from build123d import *

# Parameters (mm, degrees)
F1_DEPTH  = 18
F2_R      = 2.1
F3_DEPTH  = 25
F4_START  = -9
F2_R_2    = 4.1
F4_DEPTH  = 16
F6_START  = -9
F5_R      = 4.1
F5_R_2    = 2.1
F6_DEPTH  = 16
F7_DEPTH  = 25
F8_R      = 1
F2_W      = 8
F2_H      = 4.2
F9_DEPTH  = 1.5
F5_W      = 4.2
F5_H      = 8
F10_DEPTH = 1.5
F11_R     = 0.5


with BuildPart() as f1:
    # F0 (on Front) → F1 (new body)
    with BuildSketch(Plane.XZ):
        Polygon((-30, 10), (-30, 0), (0, 0), (21.2132034356, 21.2132034356), (14.1421356237, 28.2842712475), align=None)
    extrude(amount=F1_DEPTH)

    # F2 (on face) → F3 (cut)
    with BuildSketch(Plane(origin=(0, 0, 0), x_dir=(1, 0, 0), z_dir=(0, 0, -1))):
        with Locations((-21, 9)):
            Circle(F2_R)
    extrude(amount=-F3_DEPTH, mode=Mode.SUBTRACT)

    # F2 (on face) → F4 (cut)
    with BuildSketch(Plane(origin=(0, 0, 0), x_dir=(1, 0, 0), z_dir=(0, 0, -1)).offset(F4_START)):
        with Locations((-21, 9)):
            Circle(F2_R_2)
        with Locations((-21, 9)):
            Circle(F2_R, mode=Mode.SUBTRACT)
    extrude(amount=-F4_DEPTH, mode=Mode.SUBTRACT)

    # F5 (on face) → F6 (cut)
    with BuildSketch(Plane(origin=(0, 0, 0), x_dir=(0, 1, 0), z_dir=(0.7071067812, 0, -0.7071067812)).offset(F6_START)):
        with Locations((-9, 21)):
            Circle(F5_R)
        with Locations((-9, 21)):
            Circle(F5_R_2, mode=Mode.SUBTRACT)
    extrude(amount=-F6_DEPTH, mode=Mode.SUBTRACT)

    # F5 (on face) → F7 (cut)
    with BuildSketch(Plane(origin=(0, 0, 0), x_dir=(0, 1, 0), z_dir=(0.7071067812, 0, -0.7071067812))):
        with Locations((-9, 21)):
            Circle(F5_R_2)
    extrude(amount=-F7_DEPTH, mode=Mode.SUBTRACT)

    # F8
    f8_edges = [f1.edges().sort_by_distance(p)[0] for p in [
        (-30, -9, 0),
        (-30, -9, 10),
        (21.213203, -9, 21.213203),
        (14.142136, -9, 28.284271),
        (-25.1, -8.999972, 12.029646),
    ]]
    fillet(f8_edges, radius=F8_R)

    # F2 (on face) → F9 (join)
    with BuildSketch(Plane(origin=(0, 0, 0), x_dir=(1, 0, 0), z_dir=(0, 0, -1))):
        with Locations((-7, 9)):
            Rectangle(F2_W, F2_H)
    extrude(amount=F9_DEPTH)

    # F5 (on face) → F10 (join)
    with BuildSketch(Plane(origin=(0, 0, 0), x_dir=(0, 1, 0), z_dir=(0.7071067812, 0, -0.7071067812))):
        with Locations((-9, 7)):
            Rectangle(F5_W, F5_H)
    extrude(amount=F10_DEPTH)

    # F11
    f11_edges = [f1.edges().sort_by_distance(p)[0] for p in [
        (-7, -6.9, 0),
        (-7, -6.9, -1.5),
        (-7, -11.1, -1.5),
        (-7, -11.1, 0),
        (4.949747, -11.1, 4.949747),
        (6.010408, -11.1, 3.889087),
        (6.010408, -6.9, 3.889087),
        (4.949747, -6.9, 4.949747),
    ]]
    fillet(f11_edges, radius=F11_R)


solid = f1.part
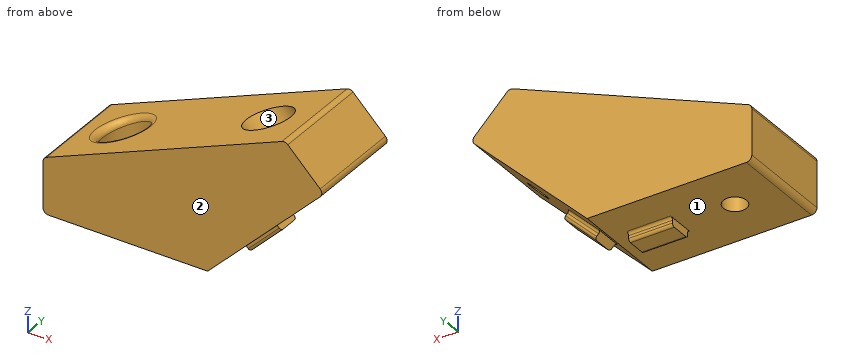
Geometry check sheet. Reference: the model listing, model coordinates, mm. Face numbers are marked on the shaded views. Give positions to 0.01 mm unless a question says otherwise; leave off trailing zeros. Loops run counter-clockwise (first coordinate to the right, second up) from the corner with the lowest first, then second, coordinate; pieces in that order, holes last. Notation, with made-up numbers: (-7.5, -20) -> (37.5, -20) arc R23 ccw to (37.5, 19) -> close; hole circle Ø10 at (80.5, -30.5). An arc over 180 degrees is marked (long way). Answer in a Markdown table with one row per item. Add a question column.
1) Cross-section at C-C on x = -1. Record the boundary of the cut face in (y, z), and give its area (3 significant figures).
2) Cross-section at A-A on z = 0.5. Record the boundary of the cut face in (x, y).
3) Gauge pin test, flat ends, axial feed: P1, Ø5.5, axis at x = -21, y = -9, coming from the -Z side; P2, Ø5, axis at x = -21, y = -9, coming from the +Z side; P3, Ø1, axis at y = -5.5, z = 23, coming from the +X side. Record the tip position at first contact, or that the pin passes through.
4) Draft check along Z on the marked faces 1, 2 and 3. Enter one of: pulls with the +Z half, pulls with the -Z half, needs draft (parallel to the pull), parting line crosses it, or undercut.
5) Material ranges on probe 1 along Y at (x, z) = (-21, 2.75); probe 2 along Y at (x, z) = (-21, 12.15); probe 3 along X at (y, z) = (-14.75, 10.25), recorded low to high. Write a range as from..to.
6) Cross-section at B-B on x = 10. State how many separate pieces and enclosed holes the cut face has, and give its area (3 significant figures).
Outcome:
| question | item | result |
|---|---|---|
| 1 | outline | (-18, 0) -> (0, 0) -> (0, 22.01) -> (-18, 22.01) -> close |
| 1 | area | 396 mm^2 |
| 2 | outline | (-29.87, -18) -> (0.5, -18) -> (0.5, 0) -> (-29.87, 0) -> close; hole circle Ø4.2 at (-21, -9) |
| 3 | P1 | stops at z = 0 |
| 3 | P2 | stops at z = 9 |
| 3 | P3 | stops at x = 19.93 |
| 4 | face 1 | pulls with the -Z half |
| 4 | face 2 | needs draft |
| 4 | face 3 | undercut |
| 5 | probe 1 | y = -18..-11.1, -6.9..0 |
| 5 | probe 2 | y = -18..-13.1, -4.9..0 |
| 5 | probe 3 | x = -29.4..10.25 |
| 6 | separate pieces | 1 |
| 6 | enclosed holes | 2 |
| 6 | area | 265 mm^2 |
